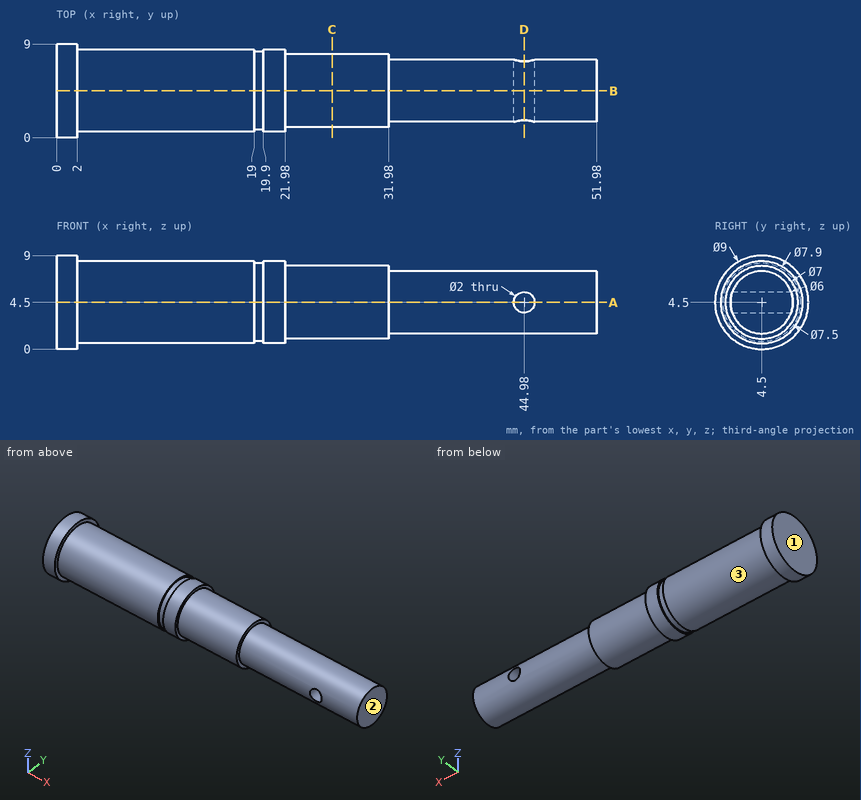
Geometry check sheet. Reference: drawing and pictorial views, mm from the part's lowest x, y, z. Round coordinates to 2 decimals unless told otherwise and drop trailing zeros. Loops run counter-clockwise (first coordinate to the right, second up) from the corner with the lowest first, then second, coordinate; pieces in that order, holes last. Notation, with made-up numbers: (5.25, 76) - (34.25, 76) arc R10 ccw to (34.25, 87) - close; hole circle Ø6 at (33, -37.5). An arc over 180 degrees is marked (long way). Use a Markdown table: item, result.
Q1. Draft check along X on the marked faces 1, 2 and 3. Enter one of: released by +X, released by -X, zero draft, split by the parting line, or undercut.
Solutions:
| item | result |
|---|---|
| face 1 | released by -X |
| face 2 | released by +X |
| face 3 | zero draft |
Q2. Go/stop test with flat-tipped pins: P1, Ø3, axis at x = 38, z = 7.5, coming from the +Y side; P2, Ø4, axis at y = 7, z = 5.5, coming from the -X side; P3, Ø1.8, axis at x = 44.98, z = 4.5, coming from the -Y side; P4, Ø2, axis at x = 25.5, z = 4, coming from the +Y side. Record where each tip stops, or that it passes through.
Solutions:
| item | result |
|---|---|
| P1 | stops at y = 7.1 |
| P2 | stops at x = 0 |
| P3 | passes through |
| P4 | stops at y = 8 |
Q3. Cross-section at A-A on z = 4.5. Record the cut outline in (x, y).
Solutions:
| item | result |
|---|---|
| outline | (0, 0) - (2, 0) - (2, 0.55) - (19, 0.55) - (19, 0.75) - (19.9, 0.75) - (19.9, 0.55) - (21.98, 0.55) - (21.98, 1) - (31.98, 1) - (31.98, 1.5) - (43.98, 1.5) - (43.98, 7.5) - (31.98, 7.5) - (31.98, 8) - (21.98, 8) - (21.98, 8.45) - (19.9, 8.45) - (19.9, 8.25) - (19, 8.25) - (19, 8.45) - (2, 8.45) - (2, 9) - (0, 9) - close; (45.98, 1.5) - (51.98, 1.5) - (51.98, 7.5) - (45.98, 7.5) - close |
Q4. Cross-section at D-D on x = 44.98. Record the cut outline in (y, z), plus the area to 3 significant figures.
Solutions:
| item | result |
|---|---|
| outline | (1.67, 3.5) arc R3 ccw to (7.33, 3.5) - close; (1.67, 5.5) - (7.33, 5.5) arc R3 ccw to start |
| area | 16.5 mm2 |
Q5. Cross-section at C-C on x = 26.5. Record the cut outline in (y, z), plus the area to 3 significant figures.
Solutions:
| item | result |
|---|---|
| outline | circle Ø7 at (4.5, 4.5) |
| area | 38.5 mm2 |
Q6. Material ranges on line 1 (X direction, y = 5.25, z = 4.5); line 2 (X direction, y = 0.75, z = 6.5); line 3 (Z direction, x = 44.98, y = 3.5), recorded low to high.
Solutions:
| item | result |
|---|---|
| line 1 | x = 0 to 43.98, 45.98 to 51.98 |
| line 2 | x = 0 to 2 |
| line 3 | z = 1.67 to 3.5, 5.5 to 7.33 |
Q7. Cross-section at B-B on y = 4.5. Record the cut outline in (x, z).
Solutions:
| item | result |
|---|---|
| outline | (0, 0) - (2, 0) - (2, 0.55) - (19, 0.55) - (19, 0.75) - (19.9, 0.75) - (19.9, 0.55) - (21.98, 0.55) - (21.98, 1) - (31.98, 1) - (31.98, 1.5) - (51.98, 1.5) - (51.98, 7.5) - (31.98, 7.5) - (31.98, 8) - (21.98, 8) - (21.98, 8.45) - (19.9, 8.45) - (19.9, 8.25) - (19, 8.25) - (19, 8.45) - (2, 8.45) - (2, 9) - (0, 9) - close; hole circle Ø2 at (44.98, 4.5) |
